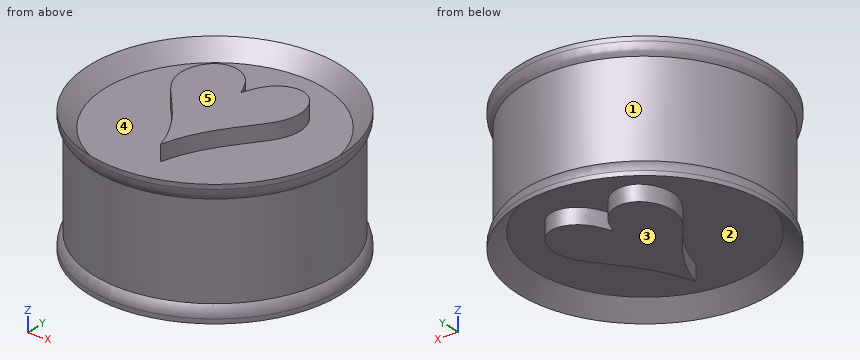
from build123d import *

# Parameters (mm, degrees)
F0_R      = 9.779
F1_DEPTH  = 7.62
F2_R      = 10.16
F2_R_2    = 8.89
F3_DEPTH  = 2.54
F5_R      = 10.16
F5_R_2    = 8.89
F6_DEPTH  = 2.54
F9_DEPTH  = 1.27
F11_DEPTH = 1.27


# Not quite as in the source:
# - a fillet or chamfer that OpenCascade refuses, or shapes differently, is made with other operations: its cross-section is extruded or revolved along the edge and cut away or added


with BuildPart() as f1:
    # F0 (on Top) → F1 (new body)
    with BuildSketch(Plane.XY):
        Circle(F0_R)
    extrude(amount=F1_DEPTH)

    # F2 (on face) → F3 (join)
    with BuildSketch(Plane.XY.offset(7.62)):
        Circle(F2_R)
        Circle(F2_R_2, mode=Mode.SUBTRACT)
    extrude(amount=F3_DEPTH)

    # F4: chamfer of 2.54 on 1 edges, made by hand


with BuildPart() as f4_tool2:
    # F4_s3 → F4_t4 (revolve)
    with BuildSketch(Plane.XZ):
        Polygon((11.43, 10.16), (8.89, 7.62), (8.89, 10.16), align=None)
    revolve(axis=Axis((0, 0, 10.16), (0, 0, 1)))

    split(bisect_by=Plane.XY.offset(7.62), keep=Keep.TOP)


with BuildPart() as f1_1:
    add(f1.part)

    # F4_t1: cut F4_tool2
    add(f4_tool2.part, mode=Mode.SUBTRACT)

    # F5 (on face) → F6 (join)
    with BuildSketch(Plane(origin=(0, 0, 0), x_dir=(1, 0, 0), z_dir=(0, 0, -1))):
        Circle(F5_R)
        Circle(F5_R_2, mode=Mode.SUBTRACT)
    extrude(amount=F6_DEPTH)

    # F7: chamfer of 2.54 on 1 edges, made by hand


with BuildPart() as f7_tool2:
    # F7_s3 → F7_t4 (revolve)
    with BuildSketch(Plane.XZ):
        Polygon((11.43, -2.54), (8.89, 0), (8.89, -2.54), align=None)
    revolve(axis=Axis((0, 0, -2.54), (0, 0, -1)))

    split(bisect_by=Plane.XY, keep=Keep.BOTTOM)


with BuildPart() as f1_2:
    add(f1_1.part)

    # F7_t1: cut F7_tool2
    add(f7_tool2.part, mode=Mode.SUBTRACT)

    # F8 (on face) → F9 (join)
    with BuildSketch(Plane.XY.offset(7.62)):
        with BuildLine():
            add(Edge.make_bspline(
                [(0, -5.8319969103), (-1.0236980804, -2.2401487669), (-4.8354001596, 0.5610413637), (-5.0054154902, 3.6583937204), (-3.9025040717, 5.331842318), (-2.2678517349, 5.574651604), (-0.814518434, 4.6455144306), (-0.3463686184, 3.5171935493), (-0.1037365128, 2.9312386094)],
                knots=[0, 0, 0, 0, 0.2996260724, 0.4641202227, 0.6025141594, 0.7280159913, 0.8588502662, 1, 1, 1, 1], degree=3))
            Line((0, -5.8319969103), (-0.1037365128, 2.9312386094))
        make_face()
        with BuildLine():
            Line((-0.1037365128, 2.9312386094), (0, -5.8319969103))
            add(Edge.make_bspline(
                [(0, -5.8319969103), (0.9383847232, -2.2169222283), (4.6827086977, 0.6737138371), (4.7793556331, 3.7742228605), (3.6371392772, 5.4210943193), (1.997197208, 5.6251399542), (0.5662657677, 4.6618597334), (0.1249568333, 3.5227729564), (-0.1037365128, 2.9312386094)],
                knots=[0, 0, 0, 0, 0.2996260724, 0.4641202227, 0.6025141594, 0.7280159913, 0.8588502662, 1, 1, 1, 1], degree=3))
        make_face()
    extrude(amount=F9_DEPTH)

    # F10 (on face) → F11 (join)
    with BuildSketch(Plane(origin=(0, 0, 0), x_dir=(1, 0, 0), z_dir=(0, 0, -1))):
        with BuildLine():
            add(Edge.make_bspline(
                [(0, 5.462912377), (1.0236980804, 1.8710642336), (4.8354001596, -0.930125897), (5.0054154902, -4.0274782537), (3.9025040717, -5.7009268513), (2.2678517349, -5.9437361373), (0.814518434, -5.0145989639), (0.3463686184, -3.8862780826), (0.1037365128, -3.3003231427)],
                knots=[0, 0, 0, 0, 0.2996260724, 0.4641202227, 0.6025141594, 0.7280159913, 0.8588502662, 1, 1, 1, 1], degree=3))
            Line((0, 5.462912377), (0.1037365128, -3.3003231427))
        make_face()
        with BuildLine():
            Line((0.1037365128, -3.3003231427), (0, 5.462912377))
            add(Edge.make_bspline(
                [(0, 5.462912377), (-0.9383847232, 1.847837695), (-4.6827086977, -1.0427983704), (-4.7793556331, -4.1433073938), (-3.6371392772, -5.7901788526), (-1.997197208, -5.9942244875), (-0.5662657677, -5.0309442667), (-0.1249568333, -3.8918574898), (0.1037365128, -3.3003231427)],
                knots=[0, 0, 0, 0, 0.2996260724, 0.4641202227, 0.6025141594, 0.7280159913, 0.8588502662, 1, 1, 1, 1], degree=3))
        make_face()
    extrude(amount=F11_DEPTH)

    # F12: fillet of radius 1.27 on 2 edges, made by hand

    # F12_s1 → F12_t2 (revolve, cut)
    with BuildSketch(Plane.XZ):
        with BuildLine():
            ThreePointArc((9.779, 0), (10.0608821461, -0.4150925255), (10.16, -0.9069614104))
            Line((10.16, -0.9069614104), (10.16, 0))
            Line((10.16, 0), (9.779, 0))
        make_face()
    revolve(axis=Axis((0, 0, 0), (0, 0, -1)), mode=Mode.SUBTRACT)

    # F12_s3 → F12_t4 (revolve, cut)
    with BuildSketch(Plane.XZ):
        with BuildLine():
            ThreePointArc((9.779, 7.62), (10.0608821461, 8.0350925255), (10.16, 8.5269614104))
            Line((10.16, 8.5269614104), (10.16, 7.62))
            Line((10.16, 7.62), (9.779, 7.62))
        make_face()
    revolve(axis=Axis((0, 0, 7.62), (0, 0, 1)), mode=Mode.SUBTRACT)


solid = f1_2.part
The model under review builds one solid part; all positions refer to its coordinate system, in mm. Face numbers are marked on the shaded views. A direction names the side the tool comes from. Coordinates: 2 decimals unless noted, no trailing zeros. Write each loop counter-clockwise with the first axis right and the second up, starting at its lowest first coordinate (ties: lowest second). Pieces come first, ordered by that corner, then holes. Notation, with made-up numbers: (31, 18) - (37, 18) arc R27 cw to (37, 56) - close; hole circle Ø11 at (-9, 23.25). An arc over 180 degrees is marked (long way). Answer as a JSON object with one key per item and string values. Group by question number.
1. Add section B-B (z = -0.25). Give the number of separate pieces and of enclosed holes in the cut face, plus the area to 3 significant figures.
2. Machinability: for the marked faces 4 and 5, which of the approach directions +Z, -Z, +X, -X, +Y, -Y give a long, thin tool a straight path to every point of the face, cutting with its end or side? Answer none if there is none.
3. To check wall thickness, follow probe 1 along X at (y, z) = (3.5, 8); probe 2 along X at (y, z) = (3, -1); probe 3 along Z at (x, y) = (7, -5). State the ranges of each line that lie inside material, in increasing order.
4. Add section A-A (z = 3.25). Give the boundary of the cut face in (x, y).
5. Mouldability with a two-part tool opening along X and no side actions: class the marked faces 1, 2 and 3 as pulls with the +X half, pulls with the -X half, needs draft (parallel to the pull), parting line crosses it, or undercut.
6. Clearance check with flat-ended pins moving along their axes: pin 1 Ø1 at (y, z) = (-4, 3) entering from -X; pin 2 Ø4 at (x, z) = (8, 0.5) entering from -Y; pin 3 Ø3 at (y, z) = (4, 7.5) entering from +X. State where each tip first meets the part, or that it passes through.
Findings:
{
 "1": {"separate pieces": "2", "enclosed holes": "1", "area": "110 mm²"},
 "2": {"face 4": "+Z", "face 5": "+Z, +X, -X, +Y, -Y"},
 "3": {"probe 1": "-9.42 to -8.58, -4.8 to -0.35, 0.12 to 4.61, 8.58 to 9.42", "probe 2": "-9.71 to -9.42, -4.66 to 4.87, 9.42 to 9.71", "probe 3": "0 to 7.62"},
 "4": {"outline": "circle Ø19.56 at (0, 0)"},
 "5": {"face 1": "parting line crosses it", "face 2": "undercut", "face 3": "needs draft"},
 "6": {"pin 1": "x = -9.13", "pin 2": "y = -7.91", "pin 3": "x = 9.76"}
}
